Can you work these out from the model? Positions are in its coordinate system, mm. A direction names the side the tool comes from. Give positions to 0.01 mm unless a question says otherwise; leave off trailing zeros. Order: outer loops, then holes, each group sorted by start corner. A loop starts at its lowest first (then second) coordinate and runs counter-clockwise, first axis right, second up. Notation, with made-up numbers: (83, -7) - (127, -7) arc R14 cw to (127, 11) - close; hole circle Ø10 at (-6.75, 21). An arc over 180 degrees is marked (long way). Return JSON: item names as keys, results as strings.
```python
from build123d import *

# Parameters (mm, degrees)
F0_R     = 12.5
F0_R_2   = 11
F1_DEPTH = 7
F2_SIZE  = 0.5
F4_R     = 2
F5_DEPTH = 4
F7_R     = 2


with BuildPart() as f1:
    # F0 (on Top) → F1 (new body)
    with BuildSketch(Plane.XY):
        Circle(F0_R)
        Circle(F0_R_2, mode=Mode.SUBTRACT)
    extrude(amount=F1_DEPTH)

    # F2
    f2_edges = [f1.edges().sort_by_distance(p)[0] for p in [
        (-11, 0, 7),
        (-12.5, 0, 7),
        (-12.5, 0, 0),
        (-11, 0, 0),
    ]]
    chamfer(f2_edges, length=F2_SIZE)

    # F4 (on offset) → F5 (join)
    with BuildSketch(Plane.YZ.offset(11)):
        with Locations((0, 3.5)):
            Circle(F4_R)
    extrude(amount=F5_DEPTH)

    # F6: F1 across plane


with BuildPart() as f1_1:
    add(f1.part)
    add(f1.part.mirror(Plane.YZ))

    # F7
    f7_edges = [f1_1.edges().sort_by_distance(p)[0] for p in [
        (-15, -2, 3.5),
        (15, -2, 3.5),
    ]]
    fillet(f7_edges, radius=F7_R)


solid = f1_1.part
```
1. Suppose I cut it at A-A (y = 0). List the corners of the cut face in (x, z) for me.
Checks:
{"outline": "(-13, 1.5) - (-12.5, 1.5) - (-12.5, 0.5) - (-12, 0) - (-11.5, 0) - (-11, 0.5) - (-11, 6.5) - (-11.5, 7) - (-12, 7) - (-12.5, 6.5) - (-12.5, 5.5) - (-13, 5.5) arc R2 ccw to start; (11, 0.5) - (11.5, 0) - (12, 0) - (12.5, 0.5) - (12.5, 1.5) - (13, 1.5) arc R2 ccw to (13, 5.5) - (12.5, 5.5) - (12.5, 6.5) - (12, 7) - (11.5, 7) - (11, 6.5) - close"}
2. Suppose I cut it at D-D (z = 6). List the corners of the cut face in (x, y) for me, plus the area to 3 significant figures.
Checks:
{"outline": "circle Ø25 at (0, 0); hole circle Ø22 at (0, 0)", "area": "111 mm^2"}
3. Suppose I cut it at C-C (x = 0). List the corners of the cut face in (y, z) for me.
Checks:
{"outline": "(-12.5, 0.5) - (-12, 0) - (-11.5, 0) - (-11, 0.5) - (-11, 6.5) - (-11.5, 7) - (-12, 7) - (-12.5, 6.5) - close; (11, 0.5) - (11.5, 0) - (12, 0) - (12.5, 0.5) - (12.5, 6.5) - (12, 7) - (11.5, 7) - (11, 6.5) - close"}
4. On a 3-axis mill with a long thin cutter (end or side, diameter ignored), from which of +Z, -Z, +X, -X, +Y, -Y can I reach the whole of each face in a straight line? I mean faces 4 (the face through (6, -10, 0)), 5 (the face through (-12.738, 1.847, 2.734)). Say none if no direction works.
Checks:
{"face 4": "-Z, +X, -X, +Y, -Y", "face 5": "-X"}
5. For pin 1 Ø2 at (y, z) = (5.5, 5.5) entering from +X; pin 2 Ø1.5 at (y, z) = (-2, 4) entering from +X; pin 3 Ø1 at (x, y) = (-10.5, -3) entering from -Z; pin 4 Ø1 at (x, y) = (-12, 7.5) entering from -Z, each with a flat end and sliding along its axis, tell me the tip position at first contact or that it passes through.
Checks:
{"pin 1": "x = 11.66", "pin 2": "x = 14.51", "pin 3": "z = 0.08", "pin 4": "through"}
6. Thinking about a two-plate mould opening in Y: for faces 1 (the face through (12.738, 1.847, 2.734)), 2 (the face through (-2.38, -10.74, 3.46)), 3 (the face through (6, -10, 7)), which applies, +Y half, -Y half, draft (parallel to the pull), parting line (faces both ways), or undercut?
Checks:
{"face 1": "parting line", "face 2": "undercut", "face 3": "draft"}
7. Suppose I cut it at B-B (z = 3.5). List the corners of the cut face in (x, y) for me, plus the area to 3 significant figures.
Checks:
{"outline": "(-13, -2) - (-12.34, -2) arc R12.5 ccw to (12.34, -2) - (13, -2) arc R2 ccw to (13, 2) - (12.34, 2) arc R12.5 ccw to (-12.34, 2) - (-13, 2) arc R2 ccw to start; hole circle Ø22 at (0, 0)", "area": "128 mm^2"}
8. If I drill on L1, parallel to Y at x = 0, z = 3.65; L2, parallel to Y at x = -8.5, z = 2.75; L3, parallel to X at y = 0, z = 2.9, over which ranges is the centre line in solid material (lowest first)? Write a range as [from, to].
Checks:
{"L1": "[-12.5, -11], [11, 12.5]", "L2": "[-9.17, -6.98], [6.98, 9.17]", "L3": "[-14.91, -11], [11, 14.91]"}
